from build123d import *

# Parameters (mm, degrees)
CROQUIS1_R                   = 10
SALIENTE_EXTRUIR1_DEPTH      = 5
SALIENTE_EXTRUIR2_DEPTH      = 10
SALIENTE_EXTRUIR2_DEPTH_BACK = 15
CROQUIS2_R                   = 2
SALIENTE_EXTRUIR3_DEPTH      = 1
REDONDEO1_R                  = 1


with BuildPart() as part:
    # Croquis1 → Saliente-Extruir1 (new body)
    with BuildSketch(Plane(origin=(0, 0, 0), x_dir=(1, 0, 0), z_dir=(0, 1, 0))):
        with Locations(Location((0, 0, 0), (0, 0, 270))):
            Circle(CROQUIS1_R)
    extrude(amount=SALIENTE_EXTRUIR1_DEPTH)

    # Croquis2 → Saliente-Extruir2 (add, two sides: drawn at the far end of the back side and taken through both)
    with BuildSketch(Plane(origin=(0, 5, 0), x_dir=(1, 0, 0), z_dir=(0, 1, 0)).offset(-SALIENTE_EXTRUIR2_DEPTH_BACK)):
        with Locations(Location((0, 0, 0), (0, 0, 270))):
            Circle(CROQUIS2_R)
    extrude(amount=SALIENTE_EXTRUIR2_DEPTH + SALIENTE_EXTRUIR2_DEPTH_BACK)

    # Croquis3 → Saliente-Extruir3 (add)
    with BuildSketch(Plane(origin=(0, 15, 0), x_dir=(1, 0, 0), z_dir=(0, 1, 0))):
        Polygon((-2.075143392, 0), (0, 7.5), (2.075143392, 0), (0, -7.5), align=None)
    extrude(amount=SALIENTE_EXTRUIR3_DEPTH)

    # Redondeo1
    redondeo1_edges = [part.edges().sort_by_distance(p)[0] for p in [
        (-2.075143392, 15.5, 0),
        (0, 15.5, 7.5),
        (2.075143392, 15.5, 0),
        (0, 15.5, -7.5),
    ]]
    fillet(redondeo1_edges, radius=REDONDEO1_R)


solid = part.part
Could you check a few things on this model? Use its own coordinates, in mm. A direction names the side the tool comes from. Give positions to 0.01 mm unless a question says otherwise; leave off trailing zeros. Order: outer loops, then holes, each group sorted by start corner. A loop starts at its lowest first (then second) coordinate and runs counter-clockwise, first axis right, second up. Notation, with made-up numbers: (52, 71.5) -> (93, 71.5) arc R8 cw to (93, 81.5) -> close; hole circle Ø7 at (67.5, 42.25). An arc over 180 degrees is marked (long way). Answer in a Markdown table with one row per item. Add a question column.
Item 1: Imagine slicing it at B-B (z = -3). List the corners of the cut face in (x, y) for me, and give its area (3 significant figures).
Item 2: Imagine slicing it at D-D (z = 8.75). List the corners of the cut face in (x, y) for me.
Item 3: Imagine slicing it at A-A (x = 0). List the corners of the cut face in (y, z) for me.
Item 4: Imagine slicing it at C-C (y = 1). List the corners of the cut face in (x, z) for me.
Item 5: Please list where these lines run through material, in increasing order: probe 1 along Z at (x, y) = (-1.75, -7.75); probe 2 along Y at (x, z) = (5, 8.25).
Item 6: We'd pull the mould along Y, two halves only. Please class faces 1 (the cylindrical face through (-2, 10, 0)), 2 (the flat face through (0, 16, 0)), 3 (the cylindrical face through (-0.02, 15.51, 4.75)), 4 (the flat face through (0, 15, -3)): pulls with the +Y half, pulls with the -Y half, needs draft (parallel to the pull), parting line crosses it, or undercut.
Item 7: I'm going to push flat-ended pins straight in: P1, Ø6, axis at y = 7.5, z = -7, coming from the +X side; P2, Ø4, axis at y = 9.5, z = -2, coming from the -X side; P3, Ø3, axis at x = -2, y = 9, coming from the -Z side. Where does each tip first touch, or does it pass through?
Item 8: For faces 5 (the cylindrical face through (-2, -5, 0)), 6 (the flat face through (-1.475, 15.493, 2.168)), 7 (the flat face through (1.475, 15.493, -2.168)), which set-ups out of +Z, -Z, +X, -X, +Y, -Y let a thin tool reach every point of the face, with its end or its side?
Result:
| question | item | result |
|---|---|---|
| 1 | outline | (-9.54, 0) -> (9.54, 0) -> (9.54, 5) -> (-9.54, 5) -> close; (-1.25, 15) -> (1.25, 15) -> (1.25, 16) -> (-1.25, 16) -> close |
| 1 | area | 97.9 mm2 |
| 2 | outline | (-4.84, 0) -> (4.84, 0) -> (4.84, 5) -> (-4.84, 5) -> close |
| 3 | outline | (-10, -2) -> (0, -2) -> (0, -10) -> (5, -10) -> (5, -2) -> (15, -2) -> (15, -4.75) -> (16, -4.75) -> (16, 4.75) -> (15, 4.75) -> (15, 2) -> (5, 2) -> (5, 10) -> (0, 10) -> (0, 2) -> (-10, 2) -> close |
| 4 | outline | circle Ø20 at (0, 0) |
| 5 | probe 1 | -0.97 to 0.97 |
| 5 | probe 2 | 0 to 5 |
| 6 | face 1 | undercut |
| 6 | face 2 | pulls with the +Y half |
| 6 | face 3 | needs draft |
| 6 | face 4 | undercut |
| 7 | P1 | x = 8.45 |
| 7 | P2 | x = -2 |
| 7 | P3 | z = -1.94 |
| 8 | face 5 | -Y |
| 8 | face 6 | +Z, -X, +Y |
| 8 | face 7 | -Z, +X, +Y |
